Autodesk Inventor part; units mm, degrees
ref_plane "YZ Plane" through (0, 0, 0) normal (1, 0, 0) x (0, 1, 0)
ref_plane "XZ Plane" through (0, 0, 0) normal (0, 1, 0) x (-1, 0, 0)
ref_plane "XY Plane" through (0, 0, 0) normal (0, 0, 1) x (1, 0, 0)
sketch "Boceto2" plane through (0, 0, 0) normal (0, 1, 0) x (-1, 0, 0)
  circle A0 centre (0, 0) radius 15
  arc A1 (-60, 0) -> (43.7033, -41.1099) centre (0, 0) ccw
  line L0 (43.7033, -41.1099) -> (120, 40)
  line L1 (120, 40) -> (120, 60)
  line L2 (120, 60) -> (-60, 60)
  line L3 (-60, 60) -> (-60, 0)
  line L4 (0, 0) -> (43.7033, -41.1099) construction
  line L5 (0, 0) -> (-60, 0) construction
  dimension "d7" = 60
  dimension "d8" = 20
  dimension "d9" = 60
  dimension "d10" = 180
  dimension "d11" = 30
extrude "Placa2" add sketch "Boceto2" along normal mid plane 14
equation "\"d7\" = h_"
equation "\"d8\" = b"
equation "\"d10\" = L"
equation "\"d11\" = hole"
equation "\"d12\" = Grosor"
equation "\"Grosor\" = epl"
equation "\"Radio_pliegue\" = Grosor"
equation "\"Anchura_desahogo_plegado\" = Grosor"
equation "\"Profundidad_desahogo_plegado\" = 0.5 * Grosor"
equation "\"Tamaño_destalonado\" = 4 * Grosor"
equation "\"Remanente_mínimo\" = 2 * Grosor"
equation "\"Radiodetransición\" = Radio_pliegue"
equation "\"Tamaño_de_radio_de_Jacobi\" = Radio_pliegue"
equation "\"TamañoSeparación\" = Grosor"
equation "\"L\" = 180"
equation "\"epl\" = 14"
equation "\"h_\" = 60"
equation "\"r\" = 60"
equation "\"hole\" = 30"
equation "\"hole_gr\" = 25.4"
equation "\"a\" = 7"
equation "\"b\" = 20"
equation "\"eb\" = 7"
equation "\"grillete\" = 0.875"
properties part number "CSM-EB-EPP-001-PL-001" material "Acero ASTM A36"
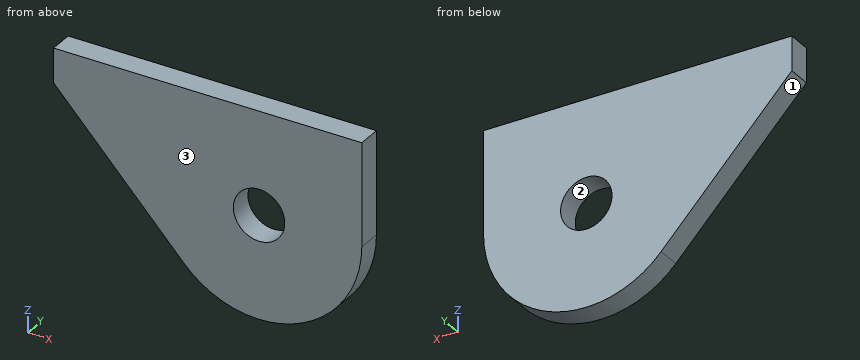
Design review of the part built by this model. Coordinates are the model's own, in mm. Face numbers are marked on the shaded views. Give positions to 0.01 mm unless a question says otherwise; leave off trailing zeros. Order: outer loops, then holes, each group sorted by start corner. A loop starts at its lowest first (then second) coordinate and runs counter-clockwise, first axis right, second up. Notation, with made-up numbers: (20, 84) - (35, 84) arc R12 ccw to (35, 105) - close; hole circle Ø11 at (80.25, 53). An arc over 180 degrees is marked (long way). Write item = value, one per line. Start each with the question number.
Q1. We need section B-B on y = 5. State the section outline as (x, z) points.
Q2. To check wall thickness, follow L1, parallel to Z at x = 0, y = 3.25; L2, parallel to Z at x = -11.5, y = 6; L3, parallel to X at y = 3.75, z = -3.5. State the ranges of each line that lie inside material, in increasing order. Write a range as from..to.
Q3. We need section D-D on x = 38. State the section outline as (y, z) points, plus the area to 3 significant figures.
Q4. We need section A-A on x = 0. State the section outline as (y, z) points, plus the area to 3 significant figures.
Q5. Mouldability with a two-part tool opening along Z and no side actions: class the marked faces 1, 2 and 3 as released by +Z, released by -Z, zero draft, split by the parting line, or undercut.
Q6. Clearance check with flat-ended pins moving along their axes: pin 1 Ø3 at (x, z) = (-13.5, 4.5) entering from +Y; pin 2 Ø1.5 at (x, y) = (-23, -1) entering from -Z; pin 3 Ø2 at (x, y) = (-89, 0) entering from -Z. State where each tip first meets the part, or that it passes through.
Q7. We need section C-C on z = 23. State the section outline as (x, y) points.
Working result:
q1.outline = (-120, 40) - (-43.7, -41.11) arc R60 ccw to (60, 0) - (60, 60) - (-120, 60) - close; hole circle Ø30 at (0, 0)
q2.L1 = -60..-15, 15..60
q2.L2 = -58.89..-9.63, 9.63..60
q2.L3 = -79.08..-14.59, 14.59..59.9
q3.outline = (-7, -46.43) - (7, -46.43) - (7, 60) - (-7, 60) - close
q3.area = 1,490 mm²
q4.outline = (-7, -60) - (7, -60) - (7, -15) - (-7, -15) - close; (-7, 15) - (7, 15) - (7, 60) - (-7, 60) - close
q4.area = 1,260 mm²
q5.face_1 = released by -Z
q5.face_2 = undercut
q5.face_3 = zero draft
q6.pin_1 = 7
q6.pin_2 = -55.72
q6.pin_3 = 5.98
q7.outline = (-104.01, -7) - (60, -7) - (60, 7) - (-104.01, 7) - close
